The model under review builds one solid part; all positions refer to its coordinate system, in mm. Face numbers are marked on the shaded views. Give positions to 0.01 mm unless a question says otherwise; leave off trailing zeros. Order: outer loops, then holes, each group sorted by start corner. A loop starts at its lowest first (then second) coordinate and runs counter-clockwise, first axis right, second up. Notation, with made-up numbers: (69, 69) - (75, 69) arc R11 cw to (75, 87) - close; hole circle Ø2 at (14, -18.75). An arc over 180 degrees is marked (long way). Put each result on its own line as item: value.
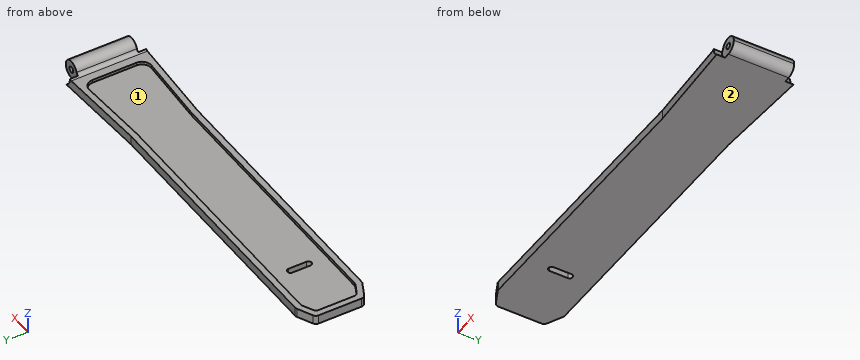
```python
from build123d import *
from OCP.BRepFilletAPI import BRepFilletAPI_MakeChamfer, BRepFilletAPI_MakeFillet

# Parameters (mm, degrees)
SALIENTE_EXTRUIR1_DEPTH = 3
CHAFL_N1_SIZE           = 6
CHAFL_N1_SIZE2          = 2.926395531
CORTAR_EXTRUIR1_DEPTH   = 1
CROQUIS8_R              = 3
SALIENTE_EXTRUIR2_DEPTH = 12.5
REDONDEO1_R             = 3
CROQUIS9_R              = 3.5
CORTAR_EXTRUIR3_DEPTH   = 3
REDONDEO2_R             = 1.5
CROQUIS10_R             = 1
CORTAR_EXTRUIR4_DEPTH   = 15
CORTAR_EXTRUIR5_DEPTH   = 96.933922834
REDONDEO3_R1            = 3
REDONDEO3_R2            = 1.5
REDONDEO4_R             = 1.5


with BuildPart() as part:
    # Croquis1 → Saliente-Extruir1 (new body)
    with BuildSketch(Plane.XY):
        Polygon((0, 11), (-95, 11), (-95, -11), (0, -11), (37, -13), (37, 13), align=None)
    extrude(amount=SALIENTE_EXTRUIR1_DEPTH)

    # Chaflán1: one chamfer whose edges measure the first distance from different faces: ONE call of the kernel's chamfer builder (chamfer() names one face for all edges)
    chafl_n1_edges_1 = [part.edges().sort_by_distance(p)[0] for p in [
        (-95, 11, 1.5),
    ]]
    chafl_n1_side_1 = [part.faces().sort_by_distance(p)[0] for p in [
        (-47.5, 11, 1.5),
    ]]
    chafl_n1_edges_2 = [part.edges().sort_by_distance(p)[0] for p in [
        (-95, -11, 1.5),
    ]]
    chafl_n1_side_2 = [part.faces().sort_by_distance(p)[0] for p in [
        (-47.5, -11, 1.5),
    ]]
    chafl_n1 = BRepFilletAPI_MakeChamfer(part.part.solid().wrapped)
    for e in chafl_n1_edges_1:
        chafl_n1.Add(CHAFL_N1_SIZE, CHAFL_N1_SIZE2, e.wrapped, chafl_n1_side_1[0].wrapped)  # the first distance lies on this face
    for e in chafl_n1_edges_2:
        chafl_n1.Add(CHAFL_N1_SIZE, CHAFL_N1_SIZE2, e.wrapped, chafl_n1_side_2[0].wrapped)  # the first distance lies on this face
    add(Compound.cast(chafl_n1.Shape()), mode=Mode.REPLACE)

    # Croquis7 → Cortar-Extruir1 (cut)
    with BuildSketch(Plane.XY.offset(3)):
        Polygon((-88.538263618, 9), (-93, 6.823865765), (-93, 0), (27, 0), (27, 10.45653975), (0.054014627, 9), align=None)
        Polygon((27, 0), (-93, 0), (-93, -6.823865765), (-88.538263618, -9), (0.054014627, -9), (27, -10.45653975), align=None)
    extrude(amount=-CORTAR_EXTRUIR1_DEPTH, mode=Mode.SUBTRACT)

    # Croquis8 → Saliente-Extruir2 (add, symmetric)
    with BuildSketch(Plane(origin=(0, 0, 0), x_dir=(1, 0, 0), z_dir=(0, 1, 0))):
        with Locations((34, -3)):
            Circle(CROQUIS8_R)
    extrude(amount=SALIENTE_EXTRUIR2_DEPTH, both=True)

    # Redondeo1
    redondeo1_edges = [part.edges().sort_by_distance(p)[0] for p in [
        (37, 0, 0),
    ]]
    fillet(redondeo1_edges, radius=REDONDEO1_R - 0.0001)  # a hair under: the kernel refuses the full size

    # Croquis9 → Cortar-Extruir3 (cut)
    with BuildSketch(Plane(origin=(0, -13, 0), x_dir=(1, 0, 0), z_dir=(0, 1, 0))):
        with Locations((34, -3)):
            Circle(CROQUIS9_R)
    cortar_extruir3 = extrude(amount=CORTAR_EXTRUIR3_DEPTH, mode=Mode.SUBTRACT)

    # Simetría1: Cortar-Extruir3 across plane
    add(cortar_extruir3.mirror(Plane.ZX), mode=Mode.SUBTRACT)

    # Redondeo2
    redondeo2_edges = [part.edges().sort_by_distance(p)[0] for p in [
        (31, 0, 3),
    ]]
    fillet(redondeo2_edges, radius=REDONDEO2_R)

    # Croquis10 → Cortar-Extruir4 (cut, symmetric)
    with BuildSketch(Plane(origin=(0, 0, 0), x_dir=(1, 0, 0), z_dir=(0, 1, 0))):
        with Locations(Location((34, -3, 0), (0, 0, 270))):
            Circle(CROQUIS10_R)
    extrude(amount=CORTAR_EXTRUIR4_DEPTH, both=True, mode=Mode.SUBTRACT)

    # Croquis11 → Cortar-Extruir5 (cut, through all)
    with BuildSketch(Plane.XY.offset(2)):
        with BuildLine():
            Line((-74, -3), (-74, 3))
            ThreePointArc((-74, 3), (-73, 4), (-72, 3))
            Line((-72, 3), (-72, -3))
            ThreePointArc((-72, -3), (-73, -4), (-74, -3))
        make_face()
    extrude(amount=-CORTAR_EXTRUIR5_DEPTH, mode=Mode.SUBTRACT)

    # Redondeo3: one fillet with a radius per group of edges: ONE call of the kernel's fillet builder (fillet() takes one radius for all edges)
    redondeo3_edges_1 = [part.edges().sort_by_distance(p)[0] for p in [
        (27, 10.45653975, 2.5),
        (27, -10.45653975, 2.5),
        (-88.538263618, 9, 2.5),
        (-88.538263618, -9, 2.5),
    ]]
    redondeo3_edges_2 = [part.edges().sort_by_distance(p)[0] for p in [
        (-93, 6.823865765, 2.5),
        (-93, -6.823865765, 2.5),
    ]]
    redondeo3 = BRepFilletAPI_MakeFillet(part.part.solid().wrapped)
    for e in redondeo3_edges_1:
        redondeo3.Add(REDONDEO3_R1, e.wrapped)
    for e in redondeo3_edges_2:
        redondeo3.Add(REDONDEO3_R2, e.wrapped)
    add(Compound.cast(redondeo3.Shape()), mode=Mode.REPLACE)

    # Redondeo4
    redondeo4_edges = [part.edges().sort_by_distance(p)[0] for p in [
        (0, 11, 1.5),
        (0, -11, 1.5),
        (-89, -11, 1.5),
        (-95, 8.073604469, 1.5),
        (-95, -8.073604469, 1.5),
        (-89, 11, 1.5),
    ]]
    fillet(redondeo4_edges, radius=REDONDEO4_R)


solid = part.part
```
(1) The part is to be moulded in two halves that separate along Y. For the marked faces 1 and 2, say which applies: pulls with the +Y half, pulls with the -Y half, needs draft (parallel to the pull), parting line crosses it, or undercut.
The answers:
face 1: undercut
face 2: needs draft
(2) Take a section at B-B, the plane x = -80.5. Write out the cut boundary in (y, z), then the cut area to 3 significant figures.
The answers:
outline: (-11, 0) - (11, 0) - (11, 3) - (9, 3) - (9, 2) - (-9, 2) - (-9, 3) - (-11, 3) - close
area: 48.0 mm^2
(3) Take a section at A-A, the plane y = 0. Count the separate pieces of the cut face and the enclosed holes in it, then the cut area to 3 significant figures.
The answers:
separate pieces: 2
enclosed holes: 1
area: 281 mm^2
(4) Clearance check with flat-ended pins moving along their axes: pin 1 Ø0.5 at (x, z) = (-38.5, 2.5) entering from +Y; pin 2 Ø1 at (y, z) = (-2.5, 4.5) entering from +X; pin 3 Ø1.5 at (x, z) = (-31.5, 1.5) entering from -Y; pin 4 Ø1.2 at (x, z) = (34, 3) entering from -Y. State where each tip first meets the part, or that it passes through.
The answers:
pin 1: y = 11
pin 2: x = 36.83
pin 3: y = -11
pin 4: through
(5) Wall thickness on L1, parallel to Y at x = -75.5, z = 2.6; L2, parallel to X at y = -3, z = 2.3; L3, parallel to Z at x = 28.5, y = 4.5: over which ranges is each line inside the solid? List them lowest first.
The answers:
L1: -11 to -9, 9 to 11
L2: -95 to -93, 27 to 33.29, 34.71 to 36.92
L3: 0 to 3
